The drawing under review shows one solid part. Ordinate dimensions are in mm from its lowest x, y, z. A direction names the side the tool comes from. Coordinates: 2 decimals unless noted, no trailing zeros. Order: outer loops, then holes, each group sorted by start corner. A loop starts at its lowest first (then second) coordinate and runs counter-clockwise, first axis right, second up. Notation, with made-up numbers: (75, -36.5) - (130, -36.5) arc R25 cw to (130, -2.5) - close; hole circle Ø7 at (54, -35). An arc over 180 degrees is marked (long way). Write item = value, one per line. Start each with the question number.
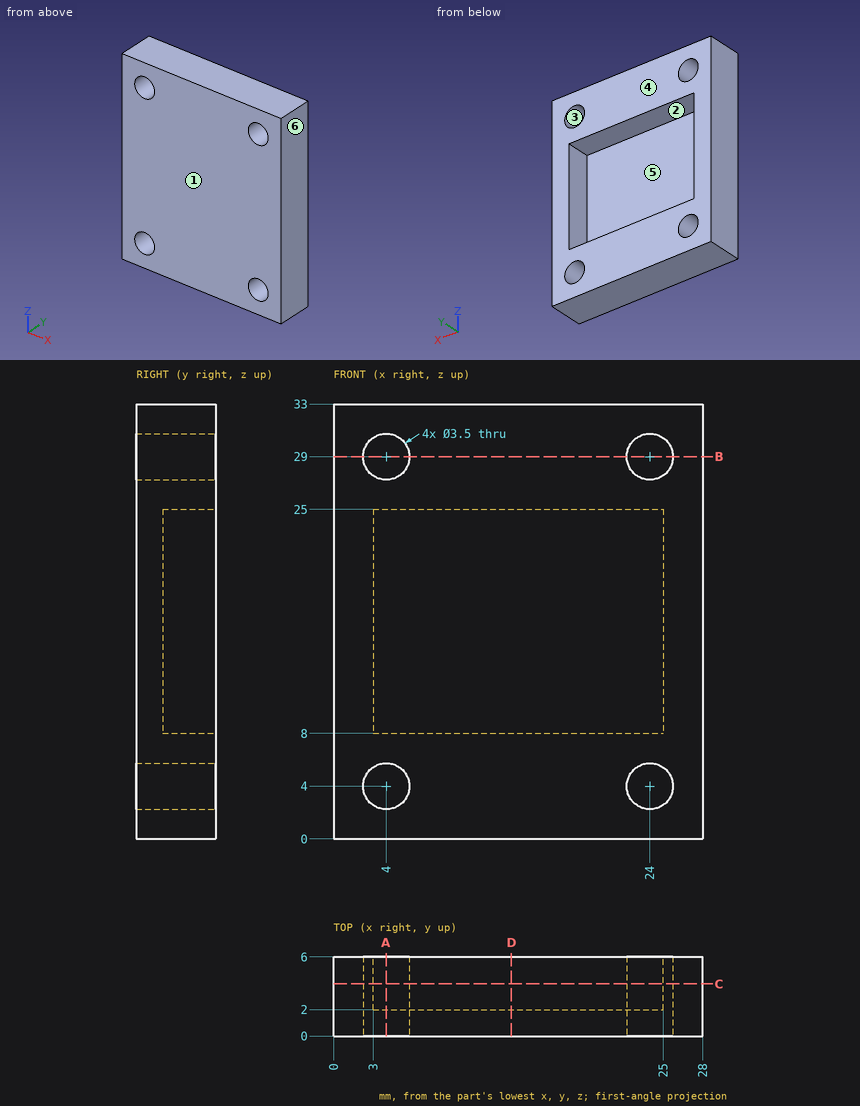
Item 1: For P1, Ø3, axis at x = 4, z = 4, coming from the +Y side (3 decimals); P2, Ø5, axis at x = 9, z = 17, coming from the +Y side, all flat-tipped, find the tip position at first contact; note any pin that passes through.
Item 2: For the marked faces 1 and 2, list the 3-axis set-ups (+Z, -Z, +X, -X, +Y, -Y) from which the entire face can be reached by the end or side of a thin tool; tool diameter is ignored.
Item 3: Add section A-A on x = 4. Give the boundary of the cut face in (y, z).
Item 4: For line 1 (X direction, y = 2, z = 4); line 2 (X direction, y = 2.4, z = 12.5); line 3 (Z direction, x = 8.25, y = 4), list the stretches that pass through material, from the lowest coordinate up.
Item 5: Add section D-D on x = 13.5. Give the boundary of the cut face in (y, z).
Item 6: Add section B-B on z = 29. Give the boundary of the cut face in (x, y).
Item 7: Add section C-C on y = 3.95. Give the boundary of the cut face in (x, z), plus the area to 3 significant figures.
Item 8: Mouldability with a two-part tool opening along X and no side actions: class the marked faces 3, 4, 5 and 6 as +X half, -X half, draft (parallel to the pull), parting line (faces both ways), or undercut.
Worked out:
q1.P1 = through
q1.P2 = 2
q2.face_1 = +Z, -Z, +X, -X, -Y
q2.face_2 = +Y
q3.outline = (0, 0) - (6, 0) - (6, 2.25) - (0, 2.25) - close; (0, 5.75) - (6, 5.75) - (6, 8) - (2, 8) - (2, 25) - (6, 25) - (6, 27.25) - (0, 27.25) - close; (0, 30.75) - (6, 30.75) - (6, 33) - (0, 33) - close
q4.line_1 = 0 to 2.25, 5.75 to 22.25, 25.75 to 28
q4.line_2 = 0 to 3, 25 to 28
q4.line_3 = 0 to 8, 25 to 33
q5.outline = (0, 0) - (6, 0) - (6, 8) - (2, 8) - (2, 25) - (6, 25) - (6, 33) - (0, 33) - close
q6.outline = (0, 0) - (2.25, 0) - (2.25, 6) - (0, 6) - close; (5.75, 0) - (22.25, 0) - (22.25, 6) - (5.75, 6) - close; (25.75, 0) - (28, 0) - (28, 6) - (25.75, 6) - close
q7.outline = (0, 0) - (28, 0) - (28, 33) - (0, 33) - close; hole circle Ø3.5 at (4, 4); hole circle Ø3.5 at (4, 29); hole (3, 8) - (25, 8) - (25, 25) - (3, 25) - close; hole circle Ø3.5 at (24, 4); hole circle Ø3.5 at (24, 29)
q7.area = 512 mm2
q8.face_3 = undercut
q8.face_4 = draft
q8.face_5 = undercut
q8.face_6 = +X half
